Geometry check sheet. Reference: the model listing, model coordinates, mm. A direction names the side the tool comes from. Coordinates: 2 decimals unless noted, no trailing zeros. Write each loop counter-clockwise with the first axis right and the second up, starting at its lowest first coordinate (ties: lowest second). Pieces come first, ordered by that corner, then holes. Notation, with made-up numbers: (-11.5, 37.5) -> (41.5, 37.5) arc R37 ccw to (41.5, 75.5) -> close; hole circle Ø8 at (17, -8.5). An arc over 180 degrees is marked (long way). Answer as CSV lines item,"result".
```python
from build123d import *

# Parameters (mm, degrees)
F0_R            = 63.5
F1_DEPTH        = 25.4
F2_R            = 45.938884012
F2_R_2          = 29.3747144419
F3_DEPTH        = 12.7
F4_R            = 3.81
F5_DEPTH        = 12.701
F5_COPIES_COUNT = 6


# Not quite as in the source:
# - a pattern or mirror of a feature is missing from the dataset's text; its kind, count and spacing are read off the source's solid


with BuildPart() as f1:
    # F0 (on Front) → F1 (new body)
    with BuildSketch(Plane.XZ):
        Circle(F0_R)
    extrude(amount=F1_DEPTH)

    # F2 (on face) → F3 (cut)
    with BuildSketch(Plane.XZ.offset(25.4)):
        Circle(F2_R)
        Circle(F2_R_2, mode=Mode.SUBTRACT)
    extrude(amount=-F3_DEPTH, mode=Mode.SUBTRACT)

    # F4 (on face) → F5 (cut, through all)
    with BuildSketch(Plane.XZ.offset(12.7)):
        with Locations((0, 38.1)):
            Circle(F4_R)
    f5 = extrude(amount=-F5_DEPTH, mode=Mode.SUBTRACT)

    # F5_copies: F5 ×6 about axis
    f5_copies_axis = Axis((0, 0, 0), (0, 1, 0))
    for i in range(1, F5_COPIES_COUNT):
        add(f5.rotate(f5_copies_axis, i * 360 / F5_COPIES_COUNT), mode=Mode.SUBTRACT)


solid = f1.part
```
Item 1: Release check for a two-part mould opening along Z. For faces 1 (the cylindrical face through (-13.77, -12.52, -61.99)), 2 (the flat face through (-1, 0, 1)), 3 (the cylindrical face through (-5.98, -19.14, 45.55)) record: +Z half, -Z half, draft (parallel to the pull), parting line (faces both ways), or undercut.
Responses:
face 1,"parting line"
face 2,"draft"
face 3,"undercut"
Item 2: Cross-section at D-D, the plane z = 0. Record the cut outline in (x, y), plus the area to 3 significant figures.
Responses:
outline,"(-63.5, -25.4) -> (-45.94, -25.4) -> (-45.94, -12.7) -> (-29.37, -12.7) -> (-29.37, -25.4) -> (29.37, -25.4) -> (29.37, -12.7) -> (45.94, -12.7) -> (45.94, -25.4) -> (63.5, -25.4) -> (63.5, 0) -> (-63.5, 0) -> close"
area,"2,810 mm2"
Item 3: Depth check by flat-ended pin: pin 1 Ø5 at (y, z) = (-20.5, -43.5) entering from +X; pin 2 Ø6 at (y, z) = (-19.5, 29) entering from -X; pin 3 Ø1 at (x, y) = (0.5, -3) entering from -Z. Enter the tip coordinate at first touch or a pass-through.
Responses:
pin 1,"stops at x = 48.49"
pin 2,"stops at x = -57.93"
pin 3,"stops at z = -63.5"
Item 4: Cross-section at A-A, the plane x = 0. Record the cut outline in (y, z).
Responses:
outline,"(-25.4, -63.5) -> (0, -63.5) -> (0, -41.91) -> (-12.7, -41.91) -> (-12.7, -45.94) -> (-25.4, -45.94) -> close; (-25.4, -29.37) -> (-12.7, -29.37) -> (-12.7, -34.29) -> (0, -34.29) -> (0, 34.29) -> (-12.7, 34.29) -> (-12.7, 29.37) -> (-25.4, 29.37) -> close; (-25.4, 45.94) -> (-12.7, 45.94) -> (-12.7, 41.91) -> (0, 41.91) -> (0, 63.5) -> (-25.4, 63.5) -> close"
Item 5: Thickness scan on probe 1 along Z at (x, y) = (0, -8); probe 2 along Z at (x, y) = (0, -18.5); probe 3 along X at (y, z) = (-18.75, -5). Record the ranges inside material, lowest first.
Responses:
probe 1,"z = -63.5 to -41.91, -34.29 to 34.29, 41.91 to 63.5"
probe 2,"z = -63.5 to -45.94, -29.37 to 29.37, 45.94 to 63.5"
probe 3,"x = -63.3 to -45.67, -28.95 to 28.95, 45.67 to 63.3"
Item 6: Cross-section at B-B, the plane z = -38.1. Record the cut outline in (x, y).
Responses:
outline,"(-50.8, -25.4) -> (-25.67, -25.4) -> (-25.67, -12.7) -> (-3.81, -12.7) -> (-3.81, 0) -> (-50.8, 0) -> close; (3.81, -12.7) -> (25.67, -12.7) -> (25.67, -25.4) -> (50.8, -25.4) -> (50.8, 0) -> (3.81, 0) -> close"
Item 7: Set-up check for faces 4 (the cylindrical face through (13.555, -19.139, -26.06)), 5 (the cylindrical face through (36.8, -6.44, 18.88)): record each of +Z, -Z, +X, -X, +Y, -Y from which the full face is reachable in a straight line by a thin tool's end or side.
Responses:
face 4,"-Y"
face 5,"+Y, -Y"
Item 8: Cross-section at C-C, the plane y = -15.75. Record the cut outline in (x, z).
Responses:
outline,"circle Ø127 at (0, 0); circle Ø58.75 at (0, 0); hole circle Ø91.88 at (0, 0)"
